Verification items for the finished model (mm, model axes). A direction names the side the tool comes from. Give positions to 0.01 mm unless a question says otherwise; leave off trailing zeros. Order: outer loops, then holes, each group sorted by start corner. A loop starts at its lowest first (then second) coordinate and runs counter-clockwise, first axis right, second up.
from build123d import *

# Parameters (mm, degrees)
CYLINDER015_R         = 2.35
CYLINDER015_DEPTH     = 33
CYLINDER016_R         = 4.35
CYLINDER016_DEPTH     = 1
CYLINDER017_R         = 4.35
CYLINDER017_DEPTH     = 1
CHAMFER003036_SIZE    = 0.85
CYLINDER021_R         = 2.5
CYLINDER021_DEPTH     = 10
CYLINDER019_R         = 2
CYLINDER019_DEPTH     = 10
CYLINDER018_R         = 2
CYLINDER018_DEPTH     = 10
CYLINDER020_R         = 2.5
CYLINDER020_DEPTH     = 10
BOX011_W              = 16
BOX011_H              = 18
BOX011_DEPTH          = 6
CYLINDER014_R         = 9
CYLINDER014_DEPTH     = 16
BOX014_W              = 4.2
BOX014_H              = 10
BOX014_DEPTH          = 22
BOX025_W              = 4.2
BOX025_H              = 10
BOX025_DEPTH          = 22
BOX013_W              = 10.2
BOX013_H              = 10
BOX013_DEPTH          = 22
CHAMFER003068003_SIZE = 1.6
BOX012_W              = 22
BOX012_H              = 23.8
BOX012_DEPTH          = 19
CHAMFER003068004_SIZE = 1
CHAMFER003068005_SIZE = 2
BOX037_W              = 5
BOX037_H              = 14
BOX037_DEPTH          = 19
CHAMFER003068011_SIZE = 3.1
CHAMFER003068012_SIZE = 0.4


with BuildPart() as cylinder015:
    # Cylinder015 → Cylinder015 (new body)
    with BuildSketch(Plane(origin=(31, 0, 6), x_dir=(0, 0, 1), z_dir=(-1, 0, 0))):
        Circle(CYLINDER015_R)
    extrude(amount=CYLINDER015_DEPTH)


with BuildPart() as cylinder016:
    # Cylinder016 → Cylinder016 (new body)
    with BuildSketch(Plane(origin=(23.15, 0, 6), x_dir=(0, 0, 1), z_dir=(-1, 0, 0))):
        Circle(CYLINDER016_R)
    extrude(amount=CYLINDER016_DEPTH)


with BuildPart() as chamfer003036:
    # Cylinder017 → Cylinder017 (new body)
    with BuildSketch(Plane(origin=(7.85, 0, 6), x_dir=(0, 0, 1), z_dir=(-1, 0, 0))):
        Circle(CYLINDER017_R)
    extrude(amount=CYLINDER017_DEPTH)

    # Fusion013005011005: union Cylinder016
    add(cylinder016.part)

    # Chamfer003036
    chamfer003036_edges = [chamfer003036.edges().sort_by_distance(p)[0] for p in [
        (7.85, 0, 1.65),
        (22.15, 0, 1.65),
    ]]
    chamfer(chamfer003036_edges, length=CHAMFER003036_SIZE)


with BuildPart() as cylinder021:
    # Cylinder021 → Cylinder021 (new body)
    with BuildSketch(Plane(origin=(15, 6.5, 3), x_dir=(1, 0, 0), z_dir=(0, 0, 1))):
        Circle(CYLINDER021_R)
    extrude(amount=CYLINDER021_DEPTH)


with BuildPart() as cylinder019:
    # Cylinder019 → Cylinder019 (new body)
    with BuildSketch(Plane(origin=(15, 6.5, 13), x_dir=(1, 0, 0), z_dir=(0, 0, 1))):
        Circle(CYLINDER019_R)
    extrude(amount=CYLINDER019_DEPTH)


with BuildPart() as fusion013005011029006008001003:
    # Cylinder018 → Cylinder018 (new body)
    with BuildSketch(Plane(origin=(15, -6.5, 13), x_dir=(1, 0, 0), z_dir=(0, 0, 1))):
        Circle(CYLINDER018_R)
    extrude(amount=CYLINDER018_DEPTH)

    # Fusion013005011029006008001003: union Cylinder019
    add(cylinder019.part)


with BuildPart() as cylinder020:
    # Cylinder020 → Cylinder020 (new body)
    with BuildSketch(Plane(origin=(15, -6.5, 3), x_dir=(1, 0, 0), z_dir=(0, 0, 1))):
        Circle(CYLINDER020_R)
    extrude(amount=CYLINDER020_DEPTH)


with BuildPart() as fusion013005011029006008001004:
    # Fusion013005011029006008001004 base: copy of Cylinder020
    add(cylinder020.part)

    # Fusion013005011029006008001004: union Cylinder021
    add(cylinder021.part)


with BuildPart() as fusion013005011029006008001005:
    # Fusion013005011029006008001005 base: copy of Cylinder020
    add(cylinder020.part)

    # Fusion013005011029006008001005: union Cylinder021, Fusion013005011029006008001003, Fusion013005011029006008001004
    add(cylinder021.part)
    add(fusion013005011029006008001003.part)
    add(fusion013005011029006008001004.part)


with BuildPart() as cube011:
    # Box011 → Box011 (new body)
    with BuildSketch(Plane(origin=(7, -9, 0), x_dir=(1, 0, 0), z_dir=(0, 0, 1))):
        with Locations((8, 9)):
            Rectangle(BOX011_W, BOX011_H)
    extrude(amount=BOX011_DEPTH)


with BuildPart() as fusion013005011004:
    # Cylinder014 → Cylinder014 (new body)
    with BuildSketch(Plane(origin=(23, 0, 6), x_dir=(0, 0, 1), z_dir=(-1, 0, 0))):
        Circle(CYLINDER014_R)
    extrude(amount=CYLINDER014_DEPTH)

    # Fusion013005011004: union Cube011
    add(cube011.part)


with BuildPart() as cube014:
    # Box014 → Box014 (new body)
    with BuildSketch(Plane(origin=(6.9, -20.3, 0), x_dir=(1, 0, 0), z_dir=(0, 0, 1))):
        with Locations((2.1, 5)):
            Rectangle(BOX014_W, BOX014_H)
    extrude(amount=BOX014_DEPTH)


with BuildPart() as cube023:
    # Box025 → Box025 (new body)
    with BuildSketch(Plane(origin=(15.9, -20.3, 0), x_dir=(1, 0, 0), z_dir=(0, 0, 1))):
        with Locations((2.1, 5)):
            Rectangle(BOX025_W, BOX025_H)
    extrude(amount=BOX025_DEPTH)


with BuildPart() as chamfer003068003:
    # Box013 → Box013 (new body)
    with BuildSketch(Plane(origin=(9.9, 10.3, 0), x_dir=(1, 0, 0), z_dir=(0, 0, 1))):
        with Locations((5.1, 5)):
            Rectangle(BOX013_W, BOX013_H)
    extrude(amount=BOX013_DEPTH)

    # Fusion013005011029006008001002: union Cube014, Cube023
    add(cube014.part)
    add(cube023.part)

    # Chamfer003068003
    chamfer003068003_edges = [chamfer003068003.edges().sort_by_distance(p)[0] for p in [
        (9.9, 10.3, 11),
        (20.1, 10.3, 11),
        (6.9, -10.3, 11),
        (11.1, -10.3, 11),
        (15.9, -10.3, 11),
        (20.1, -10.3, 11),
    ]]
    chamfer(chamfer003068003_edges, length=CHAMFER003068003_SIZE)


with BuildPart() as chamfer003068005:
    # Box012 → Box012 (new body)
    with BuildSketch(Plane(origin=(4.6, -11.9, 0), x_dir=(1, 0, 0), z_dir=(0, 0, 1))):
        with Locations((11, 11.9)):
            Rectangle(BOX012_W, BOX012_H)
    extrude(amount=BOX012_DEPTH)

    # Cut001001036003: cut Chamfer003068003
    add(chamfer003068003.part, mode=Mode.SUBTRACT)

    # Cut001001036004: cut Fusion013005011004
    add(fusion013005011004.part, mode=Mode.SUBTRACT)

    # Cut001001036005: cut Fusion013005011029006008001005
    add(fusion013005011029006008001005.part, mode=Mode.SUBTRACT)

    # Fusion013005011029006008001006: union Chamfer003036
    add(chamfer003036.part)

    # Chamfer003068004
    chamfer003068004_edges = [chamfer003068005.edges().sort_by_distance(p)[0] for p in [
        (4.6, -11.9, 9.5),
        (4.6, 11.9, 9.5),
    ]]
    chamfer(chamfer003068004_edges, length=CHAMFER003068004_SIZE)

    # Chamfer003068005
    chamfer003068005_edges = [chamfer003068005.edges().sort_by_distance(p)[0] for p in [
        (26.6, 11.9, 9.5),
        (26.6, -11.9, 9.5),
    ]]
    chamfer(chamfer003068005_edges, length=CHAMFER003068005_SIZE)


with BuildPart() as chamfer003068005_1:
    # Chamfer003068005 placement: moved
    add(chamfer003068005.part.moved(Location((0.5, 0, 0))))


with BuildPart() as chamfer003068012:
    # Box037 → Box037 (new body)
    with BuildSketch(Plane(origin=(2, -7, 0), x_dir=(1, 0, 0), z_dir=(0, 0, 1))):
        with Locations((2.5, 7)):
            Rectangle(BOX037_W, BOX037_H)
    extrude(amount=BOX037_DEPTH)

    # Chamfer003068011
    chamfer003068011_edges = [chamfer003068012.edges().sort_by_distance(p)[0] for p in [
        (2, -7, 9.5),
        (2, 7, 9.5),
    ]]
    chamfer(chamfer003068011_edges, length=CHAMFER003068011_SIZE)

    # Fusion013005011029006008001009: union Chamfer003068005
    add(chamfer003068005_1.part)

    # Cut001001036010002: cut Cylinder015
    add(cylinder015.part, mode=Mode.SUBTRACT)

    # Chamfer003068012
    chamfer003068012_edges = [chamfer003068012.edges().sort_by_distance(p)[0] for p in [
        (2, 0, 19),
        (2, 0, 0),
        (3.55, -5.45, 0),
        (3.55, -5.45, 19),
        (3.55, 5.45, 0),
        (3.55, 5.45, 19),
        (5.1, -8.95, 19),
        (5.1, -8.95, 0),
        (5.1, 8.95, 19),
        (5.1, 8.95, 0),
        (5.6, -11.4, 0),
        (5.6, -11.4, 19),
        (5.6, 11.4, 0),
        (5.6, 11.4, 19),
        (6.75, -11.9, 0),
        (6.75, -11.9, 19),
        (22.85, -11.9, 0),
        (22.85, -11.9, 19),
        (19.8, -11.1, 0),
        (19.8, -11.1, 19),
        (18.5, -10.3, 0),
        (18.5, -10.3, 19),
        (17.2, -11.1, 0),
        (17.2, -11.1, 19),
        (14, -11.9, 0),
        (14, -11.9, 19),
        (10.8, -11.1, 0),
        (10.8, -11.1, 19),
        (9.5, -10.3, 0),
        (9.5, -10.3, 19),
        (8.2, -11.1, 0),
        (8.2, -11.1, 19),
        (8.25, 11.9, 0),
        (8.25, 11.9, 19),
        (11.2, 11.1, 0),
        (11.2, 11.1, 19),
        (15.5, 10.3, 0),
        (15.5, 10.3, 19),
        (19.8, 11.1, 0),
        (19.8, 11.1, 19),
        (22.85, 11.9, 0),
        (22.85, 11.9, 19),
        (26.1, 10.9, 0),
        (26.1, 10.9, 19),
        (27.1, 0, 19),
        (27.1, 0, 0),
        (26.1, -10.9, 0),
        (26.1, -10.9, 19),
        (23.5, 0, 0),
        (15.5, 9, 0),
        (7.5, 0, 0),
        (15.5, -9, 0),
    ]]
    chamfer(chamfer003068012_edges, length=CHAMFER003068012_SIZE)


solid = chamfer003068012.part
(1) Release check for a two-part mould opening along Y. For faces 1 (the flat face through (23, 11.9, 9)), 2 (the cylindrical face through (15.6, 9, 11)), 3 (the flat face through (17.13, -10.89, 18.8)), 4 (the flat face through (2, 0, 9)) record: pulls with the +Y half, pulls with the -Y half, needs draft (parallel to the pull), parting line crosses it, or undercut.
Solved:
face 1: pulls with the +Y half
face 2: undercut
face 3: pulls with the -Y half
face 4: needs draft
(2) Section check B-B, the plane x = 12.5. Enter the section's corners in (y, z).
Solved:
outline: (-11.9, 0.4) - (-11.5, 0) - (-9.4, 0) - (-9, 0.4) - (-9, 6) arc R9 cw to (9, 6) - (9, 0.4) - (9.4, 0) - (9.9, 0) - (10.3, 0.4) - (10.3, 18.6) - (9.9, 19) - (-11.5, 19) - (-11.9, 18.6) - close
(3) Section check A-A, the plane y = 0. Give the number of separate pieces and of enclosed holes in the cut face, then the cut area to 3 significant figures.
Solved:
separate pieces: 3
enclosed holes: 0
area: 199 mm2
(4) Section check C-C, the plane y = 6.5. Enter the section's corners in (x, z).
Solved:
outline: (4.6, 0.4) - (5.17, 0) - (7.1, 0) - (7.5, 0.4) - (7.5, 12.22) - (13, 12.22) - (13, 13) - (13.5, 13) - (13.5, 19) - (5.17, 19) - (4.6, 18.6) - close; (17.5, 13) - (18, 13) - (18, 12.22) - (23.5, 12.22) - (23.5, 0.4) - (23.9, 0) - (26.7, 0) - (27.1, 0.4) - (27.1, 18.6) - (26.7, 19) - (17.5, 19) - close
(5) Set-up check for faces 5 (the flat face through (11.2, 11.1, 9.4)), 6 (the flat face through (10.8, -11.1, 9.4)), 7 (the flat face through (15, 9, 3)): record each of +Z, -Z, +X, -X, +Y, -Y from which the full face is reachable in a straight line by a thin tool's end or side.
Solved:
face 5: +Z, -Z, +Y
face 6: +Z, -Z, -Y
face 7: -Z
(6) Go/stop test with flat-tipped pins: pin 1 (4.5 mm diameter, centred on x = 15.5, y = 6.5, fed in from -Z); pin 2 (2 mm diameter, centred on y = -1, z = 5.5, fed in from -X); pin 3 (6.5 mm diameter, centred on x = 15.5, y = -6.5, fed in from -Z); pin 4 (2 mm diameter, centred on x = 18.5, z = 7.5, fed in from +Y). Record where each tip stops, or that it passes through.
Solved:
pin 1: stops at z = 13
pin 2: passes through
pin 3: stops at z = 0
pin 4: stops at y = 10.8
(7) Scan lines: line 1 (Y direction, x = 15.5, z = 15.75); line 2 (X direction, y = 2.25, z = 13.5); line 3 (Y direction, x = 22.75, z = 8.5). Record each from-to range of solid material in increasing order.
Solved:
line 1: y = -11.9 to -8.5, -4.5 to 4.5, 8.5 to 10.3
line 2: x = 2 to 7.5, 23.5 to 27.1
line 3: y = -11.9 to -8.65, -2.59 to 2.59, 8.65 to 11.9
